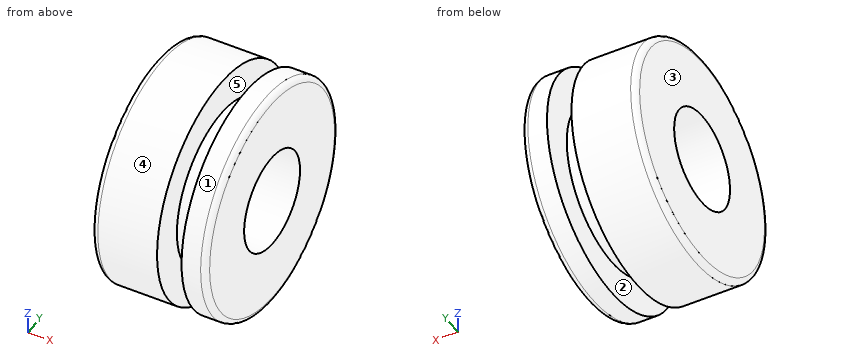
```python
from build123d import *

# Parameters (mm, degrees)
F2_R          = 17
F3_DEPTH      = 254
F3_TAPER      = -3
F3_DEPTH_BACK = 40
F4_R          = 2
F5_R          = 2


with BuildPart() as f1:
    # F0 (on Front) → F1 (revolve)
    with BuildSketch(Plane.XZ):
        Polygon((-73.0582855594, 16.432710439), (-73.0582855594, -23.567289561), (-33.0582855594, -23.567289561), (-33.0582855594, 16.432710439), (-41.7476892471, 16.432710439), (-41.7476892471, 4.3930672109), (-50.3192096949, 4.3930672109), (-50.3192096949, 16.432710439), align=None)
    revolve(axis=Axis((-53.0582855594, 0, -23.567289561), (1, 0, 0)))

    # F2 (on face) → F3 (cut, two sides)
    with BuildSketch(Plane.YZ.offset(-33.0582855594)) as f3_sk:
        with Locations((0, -23.567289561)):
            Circle(F2_R)
    extrude(amount=F3_DEPTH, taper=F3_TAPER, mode=Mode.SUBTRACT)
    extrude(f3_sk.sketch, amount=-F3_DEPTH_BACK, mode=Mode.SUBTRACT)

    # F4
    f4_edges = [f1.edges().sort_by_distance(p)[0] for p in [
        (-33.058286, 0, -63.56729),
    ]]
    fillet(f4_edges, radius=F4_R)

    # F5
    f5_edges = [f1.edges().sort_by_distance(p)[0] for p in [
        (-73.058286, 0, -63.56729),
    ]]
    fillet(f5_edges, radius=F5_R)


solid = f1.part
```
The listing builds one solid part. Answer for the finished solid, in the listing's coordinates (mm). Face numbers are marked on the shaded views. A direction names the side the tool comes from. Coordinates: 2 decimals unless noted, no trailing zeros. Loops run counter-clockwise (first coordinate to the right, second up) from the corner with the lowest first, then second, coordinate; pieces in that order, holes last. Notation, with made-up numbers: (87, 65.25) - (135, 65.25) arc R20 ccw to (135, 77.25) - close; hole circle Ø6 at (26, -12). An arc over 180 degrees is marked (long way). Write item = value, one per line.
1) Each of these flat-tipped pins is pushed along its axis until it touches: P1, Ø5, axis at x = -39, y = 13.5, coming from the +Z side; P2, Ø8, axis at x = -57.5, y = -11, coming from the +Z side; P3, Ø3, axis at x = -63, y = 11, coming from the -Z side. Where does it stop, or does it pass through?
Responses:
P1 = 14.89
P2 = 15.82
P3 = -62.42
2) Which of the six approach directions +Z, -Z, +X, -X, +Y, -Y give full straight-line access (tool end or side, diameter ignored) to the marked faces 4 and 5?
Responses:
face_4 = +X, -X
face_5 = none
3) Section A-A (y = 0) is taken. Determine the outline of the cut face in (x, z), plus the area to 3 significant figures.
Responses:
outline = (-73.06, -61.57) arc R2 ccw to (-71.06, -63.57) - (-50.32, -63.57) - (-50.32, -51.53) - (-41.75, -51.53) - (-41.75, -63.57) - (-35.06, -63.57) arc R2 ccw to (-33.06, -61.57) - (-33.06, -40.57) - (-73.06, -40.57) - close; (-73.06, -6.57) - (-33.06, -6.57) - (-33.06, 14.43) arc R2 ccw to (-35.06, 16.43) - (-41.75, 16.43) - (-41.75, 4.39) - (-50.32, 4.39) - (-50.32, 16.43) - (-71.06, 16.43) arc R2 ccw to (-73.06, 14.43) - close
area = 1,630 mm^2
4) Determine the mould class of the marked faces 1, 2 and 3 for opening direction X: pulls with the +X half, pulls with the -X half, needs draft (parallel to the pull), parting line crosses it, or undercut.
Responses:
face_1 = needs draft
face_2 = undercut
face_3 = pulls with the -X half
5) Find the intervals of material crossed by line 1 along Z through (x, y) = (-61, 0); line 2 along X through (y, z) = (13, -54); line 3 along Z through (x, y) = (-66.5, -4), in increasing order.
Responses:
line_1 = -63.57 to -40.57, -6.57 to 16.43
line_2 = -73.06 to -50.32, -41.75 to -33.06
line_3 = -63.37 to -40.09, -7.04 to 16.23
